Part model, mm, in its own coordinate system. Round coordinates to 2 decimals unless told otherwise and drop trailing zeros. Loops run counter-clockwise (first coordinate to the right, second up) from the corner with the lowest first, then second, coordinate; pieces in that order, holes last.
from build123d import *

# Parameters (mm, degrees)
SKETCH2_W           = 460.1972
SKETCH2_H           = 279.4
SKETCH2_W_2         = 42.381054546
SKETCH2_H_2         = 2.9972
SKETCH2_W_3         = 2.9972
SKETCH2_H_3         = 37.773428571
SKETCH2_H_4         = 40.770628571
BOSS_EXTRUDE1_DEPTH = 5.588
SKETCH3_W           = 2.9972
SKETCH3_H           = 40.770628572
CUT_EXTRUDE1_DEPTH  = 274.363071042
SKETCH4_W           = 497.9416
SKETCH4_H           = 317.1444
SKETCH4_W_2         = 2.2
SKETCH4_H_2         = 7.4295
SKETCH4_W_3         = 466.1916
SKETCH4_H_3         = 285.3944
BOSS_EXTRUDE2_DEPTH = 5.588


with BuildPart() as part:
    # Sketch2 → Boss-Extrude1 (new body)
    with BuildSketch(Plane(origin=(0, 0, 0), x_dir=(1, 0, 0), z_dir=(0, 1, 0))):
        Rectangle(SKETCH2_W, SKETCH2_H)
        with Locations((-169.524218182, 141.1986)):
            Rectangle(SKETCH2_W_2, SKETCH2_H_2)
        with Locations((-231.5972, 120.813285715)):
            Rectangle(SKETCH2_W_3, SKETCH2_H_3)
        with Locations((-231.5972, 40.770628572)):
            Rectangle(SKETCH2_W_3, SKETCH2_H_4)
        with Locations((-231.5972, -40.770628572)):
            Rectangle(SKETCH2_W_3, SKETCH2_H_4)
        with Locations((-84.762109091, 141.1986)):
            Rectangle(SKETCH2_W_2, SKETCH2_H_2)
        with Locations((0, 141.1986)):
            Rectangle(SKETCH2_W_2, SKETCH2_H_2)
        with Locations((84.762109091, 141.1986)):
            Rectangle(SKETCH2_W_2, SKETCH2_H_2)
        with Locations((169.524218182, 141.1986)):
            Rectangle(SKETCH2_W_2, SKETCH2_H_2)
        with Locations((169.524218182, -141.1986)):
            Rectangle(SKETCH2_W_2, SKETCH2_H_2)
        with Locations((84.762109091, -141.1986)):
            Rectangle(SKETCH2_W_2, SKETCH2_H_2)
        with Locations((0, -141.1986)):
            Rectangle(SKETCH2_W_2, SKETCH2_H_2)
        with Locations((-84.762109091, -141.1986)):
            Rectangle(SKETCH2_W_2, SKETCH2_H_2)
        with Locations((-169.524218182, -141.1986)):
            Rectangle(SKETCH2_W_2, SKETCH2_H_2)
        with Locations((-231.5972, -120.813285715)):
            Rectangle(SKETCH2_W_3, SKETCH2_H_3)
        with Locations((231.5972, -120.813285715)):
            Rectangle(SKETCH2_W_3, SKETCH2_H_3)
        with Locations((231.5972, -40.770628572)):
            Rectangle(SKETCH2_W_3, SKETCH2_H_4)
        with Locations((231.5972, 40.770628572)):
            Rectangle(SKETCH2_W_3, SKETCH2_H_4)
        with Locations((231.5972, 120.813285715)):
            Rectangle(SKETCH2_W_3, SKETCH2_H_3)
    extrude(amount=BOSS_EXTRUDE1_DEPTH)

    # Sketch3 → Cut-Extrude1 (cut, through all)
    with BuildSketch(Plane(origin=(0, 5.588, 0), x_dir=(1, 0, 0), z_dir=(0, 1, 0))):
        with Locations((50.8, -81.541257143)):
            Rectangle(SKETCH3_W, SKETCH3_H)
        with Locations((50.8, 81.541257143)):
            Rectangle(SKETCH3_W, SKETCH3_H)
    extrude(amount=-CUT_EXTRUDE1_DEPTH, mode=Mode.SUBTRACT)

    # Sketch4 → Boss-Extrude2 (add)
    with BuildSketch(Plane(origin=(0, 5.588, 0), x_dir=(1, 0, 0), z_dir=(0, 1, 0))):
        Rectangle(SKETCH4_W, SKETCH4_H)
        with Locations((-234.1958, 150.6347)):
            Rectangle(SKETCH4_W_2, SKETCH4_H_2, mode=Mode.SUBTRACT)
        Rectangle(SKETCH4_W_3, SKETCH4_H_3, mode=Mode.SUBTRACT)
        with Locations((234.1958, -150.6347)):
            Rectangle(SKETCH4_W_2, SKETCH4_H_2, mode=Mode.SUBTRACT)
        with Locations((-234.1958, -150.6347)):
            Rectangle(SKETCH4_W_2, SKETCH4_H_2, mode=Mode.SUBTRACT)
        with Locations((234.1958, 150.6347)):
            Rectangle(SKETCH4_W_2, SKETCH4_H_2, mode=Mode.SUBTRACT)
    extrude(amount=-BOSS_EXTRUDE2_DEPTH)


solid = part.part
1) Drop a flat-ended pin along its axis: pin 1 Ø5 at (x, z) = (105.5, 20) entering from -Y. Give the stop position or say it passes through.
Values:
pin 1: stops at y = 0
2) Slice it at C-C, the plane y = 1.45. Give the number of separate pieces and of enclosed holes in the cut face, then the cut area to 3 significant figures.
Values:
separate pieces: 1
enclosed holes: 24
area: 155,000 mm2
3) Wall check: line 1 along X through (y, z) = (1.3, 84.5); line 2 along X through (y, z) = (4.4, -9); line 3 along Z through (x, y) = (-199, 5.3). Give the ranges that are in metal, low to high.
Values:
line 1: x = -248.97 to -233.1, -230.1 to 49.3, 52.3 to 230.1, 233.1 to 248.97
line 2: x = -248.97 to -233.1, -230.1 to 230.1, 233.1 to 248.97
line 3: z = -158.57 to -142.7, -139.7 to 139.7, 142.7 to 158.57
4) Slice it at B-B, the plane z = -69. Give the cut face in (x, y).
Values:
outline: (-248.97, 0) - (-233.1, 0) - (-233.1, 5.59) - (-248.97, 5.59) - close; (-230.1, 0) - (49.3, 0) - (49.3, 5.59) - (-230.1, 5.59) - close; (52.3, 0) - (230.1, 0) - (230.1, 5.59) - (52.3, 5.59) - close; (233.1, 0) - (248.97, 0) - (248.97, 5.59) - (233.1, 5.59) - close
5) Slice it at A-A, the plane x = -205.5. Give the cut face in (y, z), then the cut area to 3 significant figures.
Values:
outline: (0, -158.57) - (5.59, -158.57) - (5.59, -142.7) - (0, -142.7) - close; (0, -139.7) - (5.59, -139.7) - (5.59, 139.7) - (0, 139.7) - close; (0, 142.7) - (5.59, 142.7) - (5.59, 158.57) - (0, 158.57) - close
area: 1,740 mm2
